from build123d import *

# Parameters (mm, degrees)
BOSS_EXTRUDE1_DEPTH  = 5
M5_CLEARANCE_HOLE1_D = 5.3
M5_TAPPED_HOLE1_D    = 4.2


with BuildPart() as part:
    # Sketch3 → Boss-Extrude1 (new body)
    with BuildSketch(Plane(origin=(0, 0, 0), x_dir=(-1, 0, 0), z_dir=(0, 1, 0))):
        with BuildLine():
            Line((-3.718320572, -3.342767136), (-17.618374366, 12.118930874))
            ThreePointArc((-17.618374366, 12.118930874), (-21.319064477, 14.826224184), (-25.796067121, 15.816674432))
            ThreePointArc((-25.796067121, 15.816674432), (-27.546375819, 16.558322133), (-28.269100189, 18.316528984))
            Line((-28.269100189, 18.316528984), (-28.269100189, 33.544684312))
            Line((-28.269100189, 33.544684312), (-23.269100189, 33.544684312))
            Line((-23.269100189, 33.544684312), (-22.007395686, 22.177884957))
            ThreePointArc((-22.007395686, 22.177884957), (-21.190062528, 20.590961046), (-19.522655818, 19.953688847))
            Line((-19.522655818, 19.953688847), (-11.061691266, 19.953688847))
            ThreePointArc((-11.061691266, 19.953688847), (-9.293924313, 20.685921894), (-8.561691266, 22.453688847))
            Line((-8.561691266, 22.453688847), (-8.561691266, 28.585543669))
            ThreePointArc((-8.561691266, 28.585543669), (-7.829458219, 30.353310622), (-6.061691266, 31.085543669))
            Line((-6.061691266, 31.085543669), (-3.561691266, 31.085543669))
            Line((-3.561691266, 31.085543669), (-3.561691266, 19.005709588))
            ThreePointArc((-3.561691266, 19.005709588), (-7.807339249, 10.626500654), (-0.291809826, 4.991477439))
            ThreePointArc((-0.291809826, 4.991477439), (4.624412894, -1.901264156), (-3.718320572, -3.342767136))
        make_face()
    extrude(amount=-BOSS_EXTRUDE1_DEPTH)

    # M5 Clearance Hole1 (through all)
    with Locations(Plane(origin=(0, 0, 0), x_dir=(-1, 0, 0), z_dir=(0, 1, 0))):
        with Locations((-13.951148511, 14.33057763)):
            Hole(M5_CLEARANCE_HOLE1_D / 2)

    # M5 Tapped Hole1 (through all)
    with Locations(Plane(origin=(0, 0, 0), x_dir=(-1, 0, 0), z_dir=(0, 1, 0))):
        with Locations((0, 0)):
            Hole(M5_TAPPED_HOLE1_D / 2)


solid = part.part
Geometry: final body of the model. Coordinates: model frame, mm. A direction names the side the tool comes from. Coordinates: 2 decimals unless noted, no trailing zeros. Loops run counter-clockwise (first coordinate to the right, second up) from the corner with the lowest first, then second, coordinate; pieces in that order, holes last. Notation, with made-up numbers: (44.25, -20) - (74.25, -20) arc R5 ccw to (74.25, -12) - close; hole circle Ø6 at (25.25, -28.5). An arc over 180 degrees is marked (long way). Put each result on its own line as item: value. Start each with the question number.
Q1. Cut plane D-D, the plane z = 31.5. Return loops of the section in (x, y), and give its area (3 significant figures).
Q2. Cut plane C-C, the plane y = -4.15. Return loops of the section in (x, z).
Q3. Pull-direction query (X, two-part tool) for faces 4 (the cylindrical face through (2.003, -2.535, 0.631)), 5 (the flat face through (10.57, -2.46, 4.28)), 6 (the flat face through (5, -2, 31.086)); classes: released by +X, released by -X, zero draft, split by the parting line, or undercut.
Q4. Line query: line 1 (Z direction, x = 0, y = -1); line 2 (X direction, y = -3.7, z = 23); line 3 (X direction, y = -3.1, z = 28.5). Output: solid intervals per line, ascending.
Q5. Cut plane B-B, the plane x = -1.5. Return loops of the section in (y, z), and give its area (3 significant figures).
Q6. Pin query (flat end, axial travel): pin 1 Ø4 at (x, z) = (13.95, 14.33) entering from -Y; pin 2 Ø1.5 at (x, y) = (20.5, -0.5) entering from -Z; pin 3 Ø0.8 at (x, y) = (5.5, -2.5) entering from +Z; pin 4 Ø2 at (x, y) = (18, -0.5) entering from -Z. Return the tip coordinate at first contact, or that it passes through.
Q7. Cut plane A-A, the plane z = 15. Return loops of the section in (x, y).
Q8. Set-up query: faces 1 (the cylindrical face through (9.31, -2.46, 20.67)), 2 (the flat face through (10, 0, 14)), 3 (the flat face through (3.562, -2, 25)). Return all of +Z, -Z, +X, -X, +Y, -Y with unobstructed straight access to the full face (end or side cutting, diameter ignored); none if empty.
Filled sheet:
1. outline: (23.04, -5) - (28.27, -5) - (28.27, 0) - (23.04, 0) - close
1. area: 26.1 mm²
2. outline: (0.29, 4.99) arc R5 ccw (long way) to (3.72, -3.34) - (17.62, 12.12) arc R11.16 cw to (25.8, 15.82) arc R2.5 ccw to (28.27, 18.32) - (28.27, 33.54) - (23.27, 33.54) - (22.01, 22.18) arc R2.5 cw to (19.52, 19.95) - (11.06, 19.95) arc R2.5 cw to (8.56, 22.45) - (8.56, 28.59) arc R2.5 ccw to (6.06, 31.09) - (3.56, 31.09) - (3.56, 19.01) arc R7.31 cw to start; hole circle Ø4.2 at (0, 0); hole circle Ø5.3 at (13.95, 14.33)
3. face 4: undercut
3. face 5: released by +X
3. face 6: zero draft
4. line 1: -5 to -2.1, 2.1 to 5
4. line 2: 3.56 to 8.56, 22.1 to 28.27
4. line 3: 3.56 to 8.56, 22.71 to 28.27
5. outline: (-5, -4.77) - (0, -4.77) - (0, -1.47) - (-5, -1.47) - close; (-5, 1.47) - (0, 1.47) - (0, 4.77) - (-5, 4.77) - close
5. area: 33.0 mm²
6. pin 1: through
6. pin 2: z = 13.96
6. pin 3: z = 31.09
6. pin 4: z = 11.43
7. outline: (7.48, -5) - (11.39, -5) - (11.39, 0) - (7.48, 0) - close; (16.52, -5) - (21.72, -5) - (21.72, 0) - (16.52, 0) - close
8. face 1: +Z, +Y, -Y
8. face 2: +Z, -Z, +X, -X, +Y
8. face 3: +Z, -X, +Y, -Y
